Work out the finished part from the listing and answer in its coordinate system (mm). Face numbers are marked on the shaded views. A direction names the side the tool comes from. Coordinates: 2 decimals unless noted, no trailing zeros. Order: outer loops, then holes, each group sorted by start corner. A loop starts at its lowest first (then second) coordinate and runs counter-clockwise, first axis right, second up. Notation, with made-up numbers: M 81.25,69 L 114.25,69 A12 ccw 114.25,85 Z; hole C 12,31 d2. An arc over 180 degrees is marked long. Write item = value, one per line. Start each with the question number.
Q1. Each of these flat-tipped pins is pushed along its axis until it touches: P1, Ø6, axis at x = -11, y = 6.5, coming from the +Z side; P2, Ø0.8, axis at y = 0.5, z = 63.5, coming from the -X side; P3, Ø10, axis at x = 7, z = 44, coming from the +Y side; P4, Ø0.8, axis at x = 22.5, y = 8, coming from the +Z side. Where does it stop, or does it pass through?
Q2. Straight lines are drawn through the part: line 1 along Z through (x, y) = (22.85, 12.5); line 2 along X through (y, z) = (10.25, 29.5); line 3 along Y through (x, z) = (20.5, 10). For each, find the intervals that lie inside material, in ascending order.
Q3. Find section A-A on z = 39. Give the vertices of the cut face in (x, y), and give its area (3 significant figures).
Q4. Find section B-B on y = 9. Give the vertices of the cut face in (x, z).
Q5. A tool of negligible diameter and unlimited length cuts with its end or side. For the marked faces 1 and 2, from which of +Z, -Z, +X, -X, +Y, -Y can it reach the whole face along a straight path? Write none if from no direction.
Q6. Find section C-C on x = 19.55. Give the vertices of the cut face in (y, z).
Q7. Determine the mould class of the marked faces 3, 4 and 5 for opening direction X: released by +X, released by -X, zero draft, split by the parting line, or undercut.
Q8. Find section D-D on z = 53.25. Give the vertices of the cut face in (x, y).
```python
from build123d import *

# Parameters (mm, degrees)
BASE_FLANGE1_DEPTH      = 49
SKETCH8_W               = 43.5
SKETCH8_H               = 1
BOSS_EXTRUDE1_DEPTH     = 32
SKETCH6_R               = 1.25
CUT_EXTRUDE1_DEPTH      = 10
CUT_EXTRUDE3_DEPTH      = 87.611561007
CUT_EXTRUDE3_DEPTH_BACK = 87.611561007
SKETCH9_R               = 1.5
SKETCH7_R               = 1.5
CUT_EXTRUDE2_DEPTH      = 70


# Sheet-metal steps are written as plain solids
with BuildPart() as part:
    # Sketch1 → Base-Flange1 (new, symmetric)
    with BuildSketch(Plane.XY):
        with BuildLine():
            Line((-23.25, 20), (-23.25, 1.5))
            ThreePointArc((-23.25, 1.5), (-22.810660172, 0.439339828), (-21.75, 0))
            Line((-21.75, 0), (21.75, 0))
            ThreePointArc((21.75, 0), (22.810660172, 0.439339828), (23.25, 1.5))
            Line((23.25, 1.5), (23.25, 20))
            Line((23.25, 20), (22.25, 20))
            Line((22.25, 20), (22.25, 1.5))
            ThreePointArc((22.25, 1.5), (22.103553391, 1.146446609), (21.75, 1))
            Line((21.75, 1), (-21.75, 1))
            ThreePointArc((-21.75, 1), (-22.103553391, 1.146446609), (-22.25, 1.5))
            Line((-22.25, 1.5), (-22.25, 20))
            Line((-22.25, 20), (-23.25, 20))
        make_face()
    extrude(amount=BASE_FLANGE1_DEPTH, both=True)

    # Sketch8 → Boss-Extrude1 (add)
    with BuildSketch(Plane.XY.offset(49)):
        with Locations((0, 0.5)):
            Rectangle(SKETCH8_W, SKETCH8_H)
    extrude(amount=BOSS_EXTRUDE1_DEPTH)

    # Sketch6 → Cut-Extrude1 (cut)
    with BuildSketch(Plane.XZ):
        with Locations(Location((19.55, 53.25, 0), (0, 0, 270))):
            Circle(SKETCH6_R)
        with Locations(Location((19.55, 61.75, 0), (0, 0, 270))):
            Circle(SKETCH6_R)
        with Locations(Location((-19.55, 53.25, 0), (0, 0, 270))):
            Circle(SKETCH6_R)
        with Locations(Location((-19.55, 61.75, 0), (0, 0, 270))):
            Circle(SKETCH6_R)
    extrude(amount=-CUT_EXTRUDE1_DEPTH, mode=Mode.SUBTRACT)

    # Sketch9 → Cut-Extrude3 (cut, two sides: drawn at the far end of the back side and taken through both)
    with BuildSketch(Plane(origin=(0, 0, 0), x_dir=(0, 0, -1), z_dir=(1, 0, 0)).offset(-CUT_EXTRUDE3_DEPTH_BACK)):
        with Locations((-39, 12.5)):
            Circle(SKETCH9_R)
    extrude(amount=CUT_EXTRUDE3_DEPTH + CUT_EXTRUDE3_DEPTH_BACK, mode=Mode.SUBTRACT)

    # Sketch7 → Cut-Extrude2 (cut)
    with BuildSketch(Plane(origin=(23.25, 0, 0), x_dir=(0, 0, -1), z_dir=(1, 0, 0))):
        with Locations(Location((39, 12.5, 0), (0, 0, 90))):
            Circle(SKETCH7_R)
    extrude(amount=-CUT_EXTRUDE2_DEPTH, mode=Mode.SUBTRACT)


solid = part.part
```
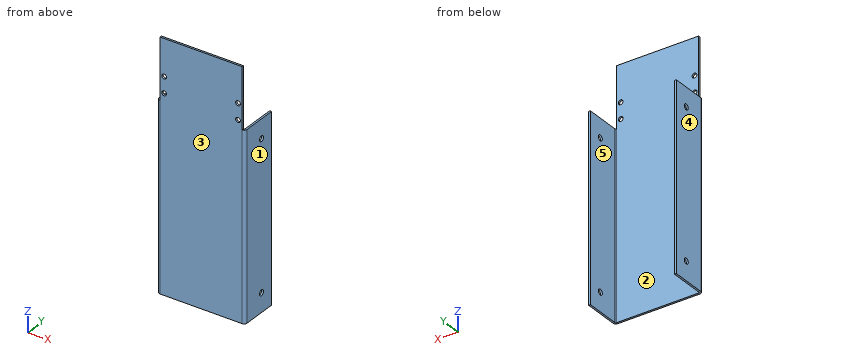
Findings below:
q1.P1 = through
q1.P2 = -21.75
q1.P3 = 1
q1.P4 = 49
q2.line_1 = -49 to -40.5, -37.5 to 37.5, 40.5 to 49
q2.line_2 = -23.25 to -22.25, 22.25 to 23.25
q2.line_3 = 0 to 1
q3.outline = M -23.25,1.5 A1.5 ccw -21.75,0 L 21.75,0 A1.5 ccw 23.25,1.5 L 23.25,11 L 22.25,11 L 22.25,1.5 A0.5 cw 21.75,1 L -21.75,1 A0.5 cw -22.25,1.5 L -22.25,11 L -23.25,11 Z; M -23.25,14 L -22.25,14 L -22.25,20 L -23.25,20 Z; M 22.25,14 L 23.25,14 L 23.25,20 L 22.25,20 Z
q3.area = 77.6 mm^2
q4.outline = M -23.25,-49 L -22.25,-49 L -22.25,49 L -23.25,49 Z; M 22.25,-49 L 23.25,-49 L 23.25,49 L 22.25,49 Z
q5.face_1 = +Z, -Z, +X, +Y, -Y
q5.face_2 = +Z, -Z, +Y
q6.outline = M 0,-49 L 1,-49 L 1,52 L 0,52 Z; M 0,54.5 L 1,54.5 L 1,60.5 L 0,60.5 Z; M 0,63 L 1,63 L 1,81 L 0,81 Z
q7.face_3 = zero draft
q7.face_4 = released by -X
q7.face_5 = undercut
q8.outline = M -21.75,0 L -20.8,0 L -20.8,1 L -21.75,1 Z; M -18.3,0 L 18.3,0 L 18.3,1 L -18.3,1 Z; M 20.8,0 L 21.75,0 L 21.75,1 L 20.8,1 Z
